Could you check a few things on this drawing? It's one solid part, dimensions in mm from its lowest x, y, z. Round coordinates to 2 decimals unless told otherwise and drop trailing zeros. Loops run counter-clockwise (first coordinate to the right, second up) from the corner with the lowest first, then second, coordinate; pieces in that order, holes last. Notation, with made-up numbers: M 75.5,-12.75 L 97.5,-12.75 A30 ccw 97.5,11.25 Z; hole C 71.25,2 d4. An arc over 180 degrees is marked long. Return JSON: item names as keys, results as strings.
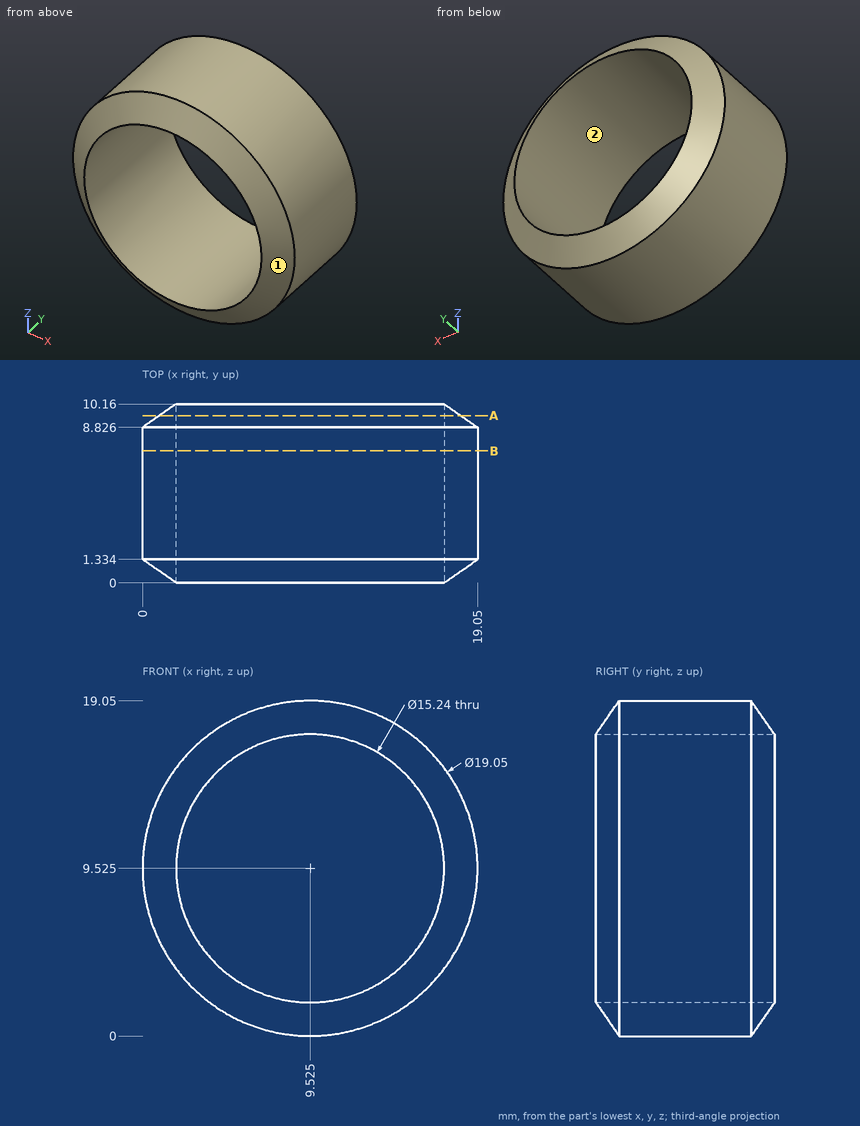
Q1. If I drill on line 1 along Z through (x, y) = (8, 4.5); line 2 along X through (y, z) = (9.5, 13.5); line 3 along Z through (x, y) = (4.5, 0.5), over which ranges is the centre line in solid material (lowest first)?
Results:
{"line 1": "z = 0.12 to 2.06, 16.99 to 18.93", "line 2": "x = 1.94 to 3.02, 16.03 to 17.11", "line 3": "z = 2.88 to 3.8, 15.25 to 16.17"}
Q2. Suppose I cut it at B-B, the plane y = 7.5. Please give me the cut outline in (x, z) (3 decimals), plus the area to 3 significant figures.
Results:
{"outline": "C 9.525,9.525 d19.05; hole C 9.525,9.525 d15.24", "area": "103 mm2"}
Q3. Suppose I cut it at A-A, the plane y = 9.5. Please give me the cut outline in (x, z) (1 decimal), plus the area to 3 significant figures.
Results:
{"outline": "C 9.5,9.5 d17.1; hole C 9.5,9.5 d15.2", "area": "47.9 mm2"}
Q4. Thinking about a two-plate mould opening in Z: for the marked faces 1 and 2, which applies, pulls with the +Z half, pulls with the -Z half, needs draft (parallel to the pull), parting line crosses it, or undercut?
Results:
{"face 1": "parting line crosses it", "face 2": "undercut"}
Q5. I'm going to push flat-ended pins straight in: pin 1 Ø5 at (y, z) = (6.5, 3) entering from -X; pin 2 Ø1 at (x, y) = (4, 3) entering from -Z; pin 3 Ø2 at (x, y) = (8, 2.5) entering from -Z. Where does each tip first touch, or does it pass through?
Results:
{"pin 1": "stops at x = 0.89", "pin 2": "stops at z = 1.43", "pin 3": "stops at z = 0.01"}
